from build123d import *

# Parameters (mm, degrees)
F0_R     = 18.034
F1_DEPTH = 34.544
F2_W     = 24.384
F2_H     = 2.286
F5_D     = 12.7
F5_DEPTH = 22.352
F5_TIP   = 3.8154649308
F7_D     = 15.875
F7_DEPTH = 22.352
F7_TIP   = 4.7693311635


# Not quite as in the source:
# - a length typed as a fraction of an inch, garbled in the dataset ("3 / 203.2 mm" for 3/8 in), is restored


with BuildPart() as f1:
    # F0 (on Right) → F1 (new body, symmetric)
    with BuildSketch(Plane.YZ):
        Circle(F0_R)
    extrude(amount=F1_DEPTH, both=True)

    # F2 (on Front) → F3 (revolve, cut)
    with BuildSketch(Plane.XZ):
        with Locations((0, 17.0634527736)):
            Rectangle(F2_W, F2_H)
    revolve(axis=Axis((6.0458816588, 0, 0), (1, 0, 0)), mode=Mode.SUBTRACT)

    # F5
    with Locations(Plane.YZ.offset(34.544)):
        with Locations((0, 0)):
            Hole(F5_D / 2, depth=F5_DEPTH)
            with Locations((0, 0, -(F5_DEPTH + F5_TIP / 2))):  # 118° drill point
                Cone(0, F5_D / 2, F5_TIP, mode=Mode.SUBTRACT)

    # F7
    with Locations(Plane(origin=(-34.544, 0, 0), x_dir=(0, -1, 0), z_dir=(-1, 0, 0))):
        with Locations((0, 0)):
            Hole(F7_D / 2, depth=F7_DEPTH)
            with Locations((0, 0, -(F7_DEPTH + F7_TIP / 2))):  # 118° drill point
                Cone(0, F7_D / 2, F7_TIP, mode=Mode.SUBTRACT)


solid = f1.part
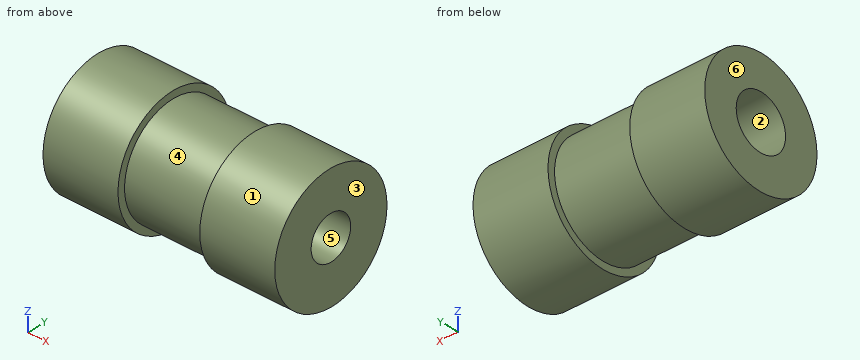
Check sheet for the modelled part. Datum: model origin and axes. Units: mm. Face numbers are marked on the shaded views. A direction names the side the tool comes from. Give positions to 0.01 mm unless a question says otherwise; leave off trailing zeros. Loops run counter-clockwise (first coordinate to the right, second up) from the corner with the lowest first, then second, coordinate; pieces in that order, holes last. Notation, with made-up numbers: M 58,6.5 L 88,6.5 A31 ccw 88,40.5 Z; hole C -17.5,14.5 d7. An arc over 180 degrees is marked long. Answer as a JSON object with one key per item and string values. Group by question number.
Q1. Cross-section at A-A on z = 11. Record the cut outline in (x, y), then the cut area to 3 significant figures.
Q2. Material ranges on line 1 along Z through (x, y) = (-23.5, 0); line 2 along Z through (x, y) = (25.75, 0); line 3 along Y through (x, z) = (-29, -0.5), recorded low to high. Write a range as [from, to].
Q3. Access from +Z, -Z, +X, -X, +Y, -Y to the whole of each face (thin tool, end or side, straight path). Record for the marked faces 4, 5 and 6.
Q4. Release check for a two-part mould opening along Y. For the marked faces 1, 2 and 3 record: released by +Y, released by -Y, zero draft, split by the parting line, or undercut.
Q5. Cross-section at B-B on y = 14. Record the cut outline in (x, z), then the cut area to 3 significant figures.
Q6. Go/stop test with flat-tipped pins: P1, Ø1, axis at y = -2, z = -5, coming from the +X side; P2, Ø1.5, axis at x = 27.5, z = 10.5, coming from the +Y side; P3, Ø1, axis at x = -10, z = 10.5, coming from the -Y side. Record where each tip stops, or that it passes through.
Evaluation:
{
 "1": {"outline": "M -34.54,-14.29 L -12.19,-14.29 L -12.19,-11.51 L 12.19,-11.51 L 12.19,-14.29 L 34.54,-14.29 L 34.54,14.29 L 12.19,14.29 L 12.19,11.51 L -12.19,11.51 L -12.19,14.29 L -34.54,14.29 Z", "area": "1,840 mm2"},
 "2": {"line 1": "z = [-18.03, -7.94], [7.94, 18.03]", "line 2": "z = [-18.03, -6.35], [6.35, 18.03]", "line 3": "y = [-18.03, -7.92], [7.92, 18.03]"},
 "3": {"face 4": "none", "face 5": "+X", "face 6": "+Z, -Z, -X, +Y, -Y"},
 "4": {"face 1": "split by the parting line", "face 2": "undercut", "face 3": "zero draft"},
 "5": {"outline": "M -34.54,-11.37 L -12.19,-11.37 L -12.19,-7.58 L 12.19,-7.58 L 12.19,-11.37 L 34.54,-11.37 L 34.54,11.37 L 12.19,11.37 L 12.19,7.58 L -12.19,7.58 L -12.19,11.37 L -34.54,11.37 Z", "area": "1,390 mm2"},
 "6": {"P1": "stops at x = 11.91", "P2": "stops at y = 15.17", "P3": "stops at y = -12.39"}
}
